Work out the finished part from the listing and answer in its coordinate system (mm). A direction names the side the tool comes from. Round coordinates to 2 decimals unless told otherwise and drop trailing zeros. Loops run counter-clockwise (first coordinate to the right, second up) from the corner with the lowest first, then second, coordinate; pieces in that order, holes last. Notation, with made-up numbers: (37, 56) -> (67, 56) arc R29 cw to (67, 84) -> close; hole circle Ø8 at (-8.75, -34.75). An arc over 180 degrees is marked (long way). Write item = value, one per line. Start each with the question number.
```python
from build123d import *

# Parameters (mm, degrees)
SKETCH1_W           = 266.7
SKETCH1_H           = 152.4
BOSS_EXTRUDE1_DEPTH = 10.16
BOSS_EXTRUDE3_DEPTH = 254
SKETCH6_W           = 482.6
SKETCH6_H           = 279.4
CUT_EXTRUDE1_DEPTH  = 6.35
LOFT1_START         = -31.75
LOFT1_DEPTH         = 63.5
BOSS_EXTRUDE4_REACH = 463.798
SKETCH7_2_W         = 63.5
SKETCH7_2_H         = 12.7
FILLET4_R           = 25.4
BOSS_EXTRUDE5_DEPTH = 2.54


# Read off the part's stored shape, not the designer's step: Loft1
with BuildPart() as part:
    # Sketch1 → Boss-Extrude1 (new body)
    with BuildSketch(Plane(origin=(0, 0, 0), x_dir=(1, 0, 0), z_dir=(0, 1, 0))):
        Rectangle(SKETCH1_W, SKETCH1_H)
    extrude(amount=BOSS_EXTRUDE1_DEPTH)

    # Loft1 outline → Loft1 (add)
    with BuildSketch(Plane.YZ.offset(LOFT1_START)):
        with BuildLine():
            Line((10.16, -19.05), (10.16, -31.75))
            add(Edge.make_bspline(
                [(10.16, -31.75), (28.965309161, -35.285855321), (52.902221104, -39.786576725), (90.992153833, -42.855395332), (120.526662629, -43.520710588), (158.632305833, -41.305063295), (187.826991891, -37.239656645), (225.166907406, -29.818418758), (248.281057243, -22.646287688), (266.440292521, -17.011625957)],
                knots=[0, 0, 0, 0, 0.219947035, 0.279966299, 0.439970653, 0.559991905, 0.720003625, 0.780025652, 1, 1, 1, 1], degree=3))
            Line((266.440292521, -17.011625957), (253.788619855, -15.904748024))
            add(Edge.make_bspline(
                [(10.16, -19.05), (27.75631541, -23.030622259), (50.154322743, -28.097478842), (85.975275474, -32.459987698), (113.853351235, -34.286596432), (150.017339583, -33.849624359), (177.910203308, -31.332603381), (213.761877453, -26.061191443), (236.17787553, -20.373323721), (253.788619855, -15.904748024)],
                knots=[0, 0, 0, 0, 0.219947035, 0.279966299, 0.439970653, 0.559991905, 0.720003625, 0.780025652, 1, 1, 1, 1], degree=3))
        make_face()
    extrude(amount=LOFT1_DEPTH)


with BuildPart() as body_2:
    # Sketch5 → Boss-Extrude3 (new, symmetric)
    with BuildSketch(Plane(origin=(0, 0, 0), x_dir=(0, 0, -1), z_dir=(1, 0, 0))):
        with BuildLine():
            Line((-38.1, 73.66), (-25.448327334, 72.553122067))
            add(Edge.make_bspline(
                [(1.116743055, 376.193266045), (38.440898524, 219.945682325), (-25.448327334, 72.553122067)],
                knots=[0, 0, 0, 1, 1, 1], degree=2))
            Line((1.116743055, 376.193266045), (-11.534929611, 377.300143978))
            Line((-11.534929611, 377.300143978), (-38.1, 73.66))
        make_face()
    extrude(amount=BOSS_EXTRUDE3_DEPTH, both=True)

    # Sketch6 → Cut-Extrude1 (cut)
    with BuildSketch(Plane(origin=(0, 3.867528241, 44.206050078), x_dir=(1, 0, 0), z_dir=(0, 0.08715574274765818, 0.9961946980917455))):
        with Locations((0, 222.459067663)):
            Rectangle(SKETCH6_W, SKETCH6_H)
    extrude(amount=-CUT_EXTRUDE1_DEPTH, mode=Mode.SUBTRACT)

    # Sketch7<2> → Boss-Extrude4 (add, up to next)
    with BuildSketch(Plane(origin=(0, 0.546894442, 6.251032081), x_dir=(1, 0, 0), z_dir=(0, 0.08715574274765883, 0.9961946980917455)), mode=Mode.PRIVATE) as boss_extrude4_sk1:
        with Locations((0, 260.559067663)):
            Rectangle(SKETCH7_2_W, SKETCH7_2_H)
    boss_extrude4_tool1 = extrude(boss_extrude4_sk1.sketch, amount=BOSS_EXTRUDE4_REACH, mode=Mode.PRIVATE) - body_2.part

    add(part.part)  # Boss-Extrude4 merges part
    add(boss_extrude4_tool1.solids().sort_by_distance((0, 260.114456, -16.458187))[0])

    # Fillet4
    fillet4_edges = [body_2.edges().sort_by_distance(p)[0] for p in [
        (133.35, 5.08, 76.2),
        (133.35, 5.08, -76.2),
        (-133.35, 5.08, -76.2),
        (-133.35, 5.08, 76.2),
    ]]
    fillet(fillet4_edges, radius=FILLET4_R)

    # Sketch9 → Boss-Extrude5 (add)
    # profile 1 of 4: a face of its own
    with BuildSketch(Plane(origin=(0, 3.867528241, 44.206050078), x_dir=(1, 0, 0), z_dir=(0, 0.08715574274765818, 0.9961946980917455))):
        with BuildLine():
            Line((-11.845192308, 80.642400996), (-10.169709869, 80.642400996))
            add(Edge.make_bspline(
                [(-10.169709869, 80.642400996), (-10.039086742, 80.641487896), (-9.786590759, 80.639722862), (-9.420774033, 80.619835181), (-9.080611029, 80.58924934), (-8.76588247, 80.547172972), (-8.477233602, 80.491494415), (-8.215036632, 80.421656578), (-7.978411563, 80.341040413), (-7.76476385, 80.246179137), (-7.569724038, 80.13558031), (-7.384527512, 80.012382096), (-7.2095379, 79.872071384), (-7.042299501, 79.717355048), (-6.884970561, 79.545402599), (-6.73493099, 79.359062194), (-6.595854438, 79.155631639), (-6.46353692, 78.939988558), (-6.343873333, 78.711219076), (-6.23949828, 78.47127043), (-6.152062666, 78.221686781), (-6.081016701, 77.962202136), (-6.024384868, 77.693677905), (-5.984760716, 77.415572233), (-5.96026467, 77.128142598), (-5.957779751, 76.933337422), (-5.956517094, 76.83435145)],
                knots=[0, 0, 0, 0, 1.44355588, 2.790409838, 4.047694926, 5.217575253, 6.298404546, 7.294384826, 8.214239204, 9.058592145, 9.873746385, 10.689560431, 11.514393297, 12.350027578, 13.205127629, 14.088021785, 14.991911688, 15.926770944, 16.882954281, 17.842803888, 18.816321264, 19.80318086, 20.814351908, 21.847355356, 22.906180909, 24, 24, 24, 24], degree=3))
            add(Edge.make_bspline(
                [(-5.956517094, 76.83435145), (-5.959823412, 76.694675801), (-5.966332092, 76.419716111), (-6.021157576, 76.016215932), (-6.109828948, 75.629420767), (-6.23450895, 75.262356277), (-6.389078777, 74.918291224), (-6.573729744, 74.603293052), (-6.785754438, 74.319052512), (-7.022682758, 74.066984889), (-7.279218425, 73.85032935), (-7.545810714, 73.664779736), (-7.825056719, 73.518458383), (-8.071111475, 73.425668764), (-8.284471646, 73.367961649), (-8.471799567, 73.333856188), (-8.684584973, 73.302579424), (-8.924811901, 73.278409413), (-9.191426528, 73.256855703), (-9.485491584, 73.245144256), (-9.80605497, 73.235413782), (-10.028716551, 73.234528126), (-10.14448117, 73.234067663)],
                knots=[0, 0, 0, 0, 1.315458931, 2.589557908, 3.828601765, 5.048913369, 6.235739168, 7.376350998, 8.481830359, 9.569842114, 10.627874879, 11.640079404, 12.624025415, 13.590060155, 14.111227486, 14.704434459, 15.382649715, 16.137166398, 16.978595427, 17.902333227, 18.909396075, 20, 20, 20, 20], degree=3))
            Line((-10.14448117, 73.234067663), (-11.845192308, 73.234067663))
            Line((-11.845192308, 73.234067663), (-11.845192308, 80.642400996))
        make_face()
        with BuildLine():
            Line((-10.515491453, 79.312700141), (-10.515491453, 74.563768517))
            Line((-10.515491453, 74.563768517), (-9.820960203, 74.563768517))
            add(Edge.make_bspline(
                [(-9.820960203, 74.563768517), (-9.738321651, 74.563919946), (-9.579380204, 74.564211192), (-9.349904733, 74.578083516), (-9.137698107, 74.592007503), (-8.943344483, 74.618435698), (-8.765429413, 74.647874846), (-8.606396987, 74.688843453), (-8.462968854, 74.731877503), (-8.336896961, 74.786665183), (-8.221425379, 74.848332363), (-8.114511884, 74.920582613), (-8.011310428, 75.000813792), (-7.913750445, 75.091385611), (-7.821462695, 75.19109873), (-7.734993209, 75.300466927), (-7.65318785, 75.419156515), (-7.578146405, 75.547795036), (-7.509573132, 75.685024038), (-7.448740954, 75.829514259), (-7.398302102, 75.982468991), (-7.356380416, 76.142456392), (-7.326422619, 76.310869336), (-7.301638255, 76.486460411), (-7.288861193, 76.669925294), (-7.287107621, 76.794760931), (-7.286217949, 76.858096108)],
                knots=[0, 0, 0, 0, 1.50275155, 2.890291501, 4.180787663, 5.369391935, 6.45668281, 7.458360028, 8.354766181, 9.177074746, 9.954075863, 10.732690366, 11.5210699, 12.329727389, 13.151100085, 13.990027547, 14.863562427, 15.770965086, 16.696477834, 17.652329173, 18.619756807, 19.62365428, 20.657822005, 21.729286259, 22.847956731, 24, 24, 24, 24], degree=3))
            add(Edge.make_bspline(
                [(-7.286217949, 76.858096108), (-7.287989874, 76.955151279), (-7.29144499, 77.144401343), (-7.324765386, 77.420048191), (-7.379004633, 77.679610993), (-7.456398814, 77.922126441), (-7.553956576, 78.14827613), (-7.676072858, 78.356144094), (-7.817492245, 78.549222228), (-7.929322837, 78.662488057), (-7.985201322, 78.719083688)],
                knots=[0, 0, 0, 0, 1.13821349, 2.219428113, 3.251817212, 4.244760574, 5.201143372, 6.134805572, 7.068016741, 8, 8, 8, 8], degree=3))
            add(Edge.make_bspline(
                [(-7.985201322, 78.719083688), (-8.0403028, 78.767310817), (-8.152841329, 78.865809267), (-8.350422003, 78.9838356), (-8.568145674, 79.087533301), (-8.810993205, 79.169754014), (-9.076617583, 79.234777659), (-9.366600873, 79.279622877), (-9.679390151, 79.308439938), (-9.896083274, 79.31124965), (-10.007949386, 79.312700141)],
                knots=[0, 0, 0, 0, 0.813307809, 1.661089106, 2.549956539, 3.493439533, 4.508053171, 5.589449661, 6.755572447, 8, 8, 8, 8], degree=3))
            Line((-10.007949386, 79.312700141), (-10.515491453, 79.312700141))
        make_face(mode=Mode.SUBTRACT)
    # profile 2 of 4: a face of its own
    with BuildSketch(Plane(origin=(0, 3.867528241, 44.206050078), x_dir=(1, 0, 0), z_dir=(0, 0.08715574274765818, 0.9961946980917455))):
        Polygon((-4.626816239, 80.642400996), (-0.637713675, 80.642400996), (-0.637713675, 79.312700141), (-3.297115385, 79.312700141), (-3.297115385, 77.888020654), (-0.637713675, 77.888020654), (-0.637713675, 76.5583198), (-3.297115385, 76.5583198), (-3.297115385, 74.563768517), (-0.637713675, 74.563768517), (-0.637713675, 73.234067663), (-4.626816239, 73.234067663), align=None)
    # profile 3 of 4: a face of its own
    with BuildSketch(Plane(origin=(0, 3.867528241, 44.206050078), x_dir=(1, 0, 0), z_dir=(0, 0.08715574274765818, 0.9961946980917455))):
        Polygon((0.691987179, 80.642400996), (2.021688034, 80.642400996), (2.021688034, 74.563768517), (4.111217949, 74.563768517), (4.111217949, 73.234067663), (0.691987179, 73.234067663), align=None)
    # profile 4 of 4: a face of its own
    with BuildSketch(Plane(origin=(0, 3.867528241, 44.206050078), x_dir=(1, 0, 0), z_dir=(0, 0.08715574274765818, 0.9961946980917455))):
        Polygon((5.250961538, 80.642400996), (6.580662393, 80.642400996), (6.580662393, 74.563768517), (8.670192308, 74.563768517), (8.670192308, 73.234067663), (5.250961538, 73.234067663), align=None)
    extrude(amount=BOSS_EXTRUDE5_DEPTH)


solid = body_2.part
```
Item 1: Flat-ended cylindrical pins translate along their axes: pin 1 (0.7 mm diameter, centred on y = 79, z = 38.5, fed in from +X); pin 2 (12 mm diameter, centred on x = 108, z = 46.5, fed in from +Y); pin 3 (0.8 mm diameter, centred on y = 77.5, z = 38.5, fed in from +X). Find the tip coordinate at first contact, or state that the pin passes through.
Item 2: The mould has two halves that part along Y. Classify faces 4 (the flat face through (-2, 0, -1)), 5 (the flat face through (3.556, 73.114, 31.863)), 6 (the flat face through (133.35, 5, 1)): pulls with the +Y half, pulls with the -Y half, needs draft (parallel to the pull), parting line crosses it, or undercut.
Item 3: Find the intervals of material crossed by line 1 along Y through (x, z) = (1, -68.5); line 2 along Z through (x, y) = (26.5, 78); line 3 along X through (y, z) = (250, -20), in increasing order. Write a range as [from, to].
Item 4: Section A-A (z = -58) is taken. Determine the outline of the cut face in (x, y), then the cut area to 3 significant figures.
Item 5: A tool of negligible diameter and unlimited length cuts with its end or side. For faces 1 (the flat face through (-133.35, 5, 1)), 2 (the flat face through (-31.75, 117, -35)), 3 (the flat face through (-241.3, 223, 22)), from which of +Z, -Z, +X, -X, +Y, -Y can it reach the whole face along a straight path? Write none if from no direction.
Worked answers:
q1.pin_1 = 6.58
q1.pin_2 = 10.16
q1.pin_3 = 8.67
q2.face_4 = pulls with the -Y half
q2.face_5 = undercut
q2.face_6 = needs draft
q3.line_1 = [0, 10.16]
q3.line_2 = [-41.78, -31.41], [23.12, 37.72]
q3.line_3 = [-31.75, 31.75]
q4.outline = (-132.31, 0) -> (132.31, 0) -> (132.31, 10.16) -> (-132.31, 10.16) -> close
q4.area = 2,690 mm2
q5.face_1 = +Z, -Z, -X, -Y
q5.face_2 = -Z, -X, +Y
q5.face_3 = +Z
